```python
from build123d import *

# Parameters (mm, degrees)
SKETCH1_R           = 18
SKETCH1_R_2         = 2.1
SKETCH1_W           = 10.3
SKETCH1_H           = 10.3
BOSS_EXTRUDE1_DEPTH = 57
CUT_EXTRUDE4_DEPTH  = 40
SKETCH6_R           = 1.5
CUT_EXTRUDE5_DEPTH  = 36
SKETCH7_R           = 3
CUT_EXTRUDE6_DEPTH  = 3
CUT_EXTRUDE7_DEPTH  = 4
CHAMFER1_SIZE       = 1
CHAMFER1_SIZE2      = 2.747477419
CUT_EXTRUDE9_DEPTH  = 6
CHAMFER2_SIZE       = 0.5
CHAMFER2_SIZE2      = 1.37373871
CUT_EXTRUDE10_DEPTH = 35
CUT_EXTRUDE11_DEPTH = 58
CHAMFER3_SIZE       = 0.5
CHAMFER3_SIZE2      = 1.37373871
CUT_EXTRUDE13_DEPTH = 2


with BuildPart() as part:
    # Sketch1 → Boss-Extrude1 (new body)
    with BuildSketch(Plane(origin=(0, 0, 0), x_dir=(1, 0, 0), z_dir=(0, 1, 0))):
        Circle(SKETCH1_R)
        with Locations((13, 0)):
            Circle(SKETCH1_R_2, mode=Mode.SUBTRACT)
        with Locations((-13, 0)):
            Circle(SKETCH1_R_2, mode=Mode.SUBTRACT)
        Rectangle(SKETCH1_W, SKETCH1_H, mode=Mode.SUBTRACT)
    extrude(amount=BOSS_EXTRUDE1_DEPTH)

    # Sketch5 → Cut-Extrude4 (cut)
    with BuildSketch(Plane(origin=(0, 57, 0), x_dir=(1, 0, 0), z_dir=(0, 1, 0))):
        with BuildLine():
            Line((5.916079783, 17), (-5.916079783, 17))
            ThreePointArc((-5.916079783, 17), (0, 18), (5.916079783, 17))
        make_face()
        with BuildLine():
            Line((5.916079783, -17), (-5.916079783, -17))
            ThreePointArc((-5.916079783, -17), (0, -18), (5.916079783, -17))
        make_face()
    extrude(amount=-CUT_EXTRUDE4_DEPTH, mode=Mode.SUBTRACT)

    # Sketch6 → Cut-Extrude5 (cut, through all)
    with BuildSketch(Plane(origin=(0, 0, -17), x_dir=(-1, 0, 0), z_dir=(0, 0, -1))):
        with Locations((0, 47)):
            Circle(SKETCH6_R)
        with Locations((0, 22)):
            Circle(SKETCH6_R)
    extrude(amount=-CUT_EXTRUDE5_DEPTH, mode=Mode.SUBTRACT)

    # Sketch7 → Cut-Extrude6 (cut)
    with BuildSketch(Plane(origin=(0, 0, -17), x_dir=(-1, 0, 0), z_dir=(0, 0, -1))):
        with Locations((0, 47)):
            Circle(SKETCH7_R)
        with Locations((0, 22)):
            Circle(SKETCH7_R)
    extrude(amount=-CUT_EXTRUDE6_DEPTH, mode=Mode.SUBTRACT)

    # Sketch8 → Cut-Extrude7 (cut)
    with BuildSketch(Plane.XY.offset(17)):
        Polygon((0, 43.8), (2.771281292, 45.4), (2.771281292, 48.6), (0, 50.2), (-2.771281292, 48.6), (-2.771281292, 45.4), align=None)
        Polygon((0, 18.8), (2.771281292, 20.4), (2.771281292, 23.6), (0, 25.2), (-2.771281292, 23.6), (-2.771281292, 20.4), align=None)
    extrude(amount=-CUT_EXTRUDE7_DEPTH, mode=Mode.SUBTRACT)

    # Chamfer1
    chamfer1_edges = [part.edges().sort_by_distance(p)[0] for p in [
        (0, 57, -5.15),
        (-5.15, 57, 0),
        (0, 57, 5.15),
        (5.15, 57, 0),
    ]]
    chamfer1_side = [part.faces().sort_by_distance(p)[0] for p in [
        (14.267618119, 57, 10.141691708),
    ]]
    chamfer(chamfer1_edges, length=CHAMFER1_SIZE, length2=CHAMFER1_SIZE2, reference=chamfer1_side[0])

    # Sketch9 → Cut-Extrude9 (cut)
    with BuildSketch(Plane.XZ):
        with BuildLine():
            Line((15.438263477, -3.358179747), (9.406640719, -2.076118753))
            ThreePointArc((9.406640719, -2.076118753), (13.862833517, 4.059312543), (15.438263477, -3.358179747))
        make_face()
        with BuildLine():
            Line((-9.458796565, -2.163880365), (-15.354920877, -3.417140276))
            ThreePointArc((-15.354920877, -3.417140276), (-13.862833517, 4.059312543), (-9.458796565, -2.163880365))
        make_face()
    extrude(amount=-CUT_EXTRUDE9_DEPTH, mode=Mode.SUBTRACT)

    # Chamfer2
    chamfer2_edges = [part.edges().sort_by_distance(p)[0] for p in [
        (13.862833517, 0, 4.059312543),
        (12.422452098, 0, -2.71714925),
        (-13.862833517, 0, 4.059312543),
        (-12.406858721, 0, -2.79051032),
    ]]
    chamfer2_side = [part.faces().sort_by_distance(p)[0] for p in [
        (-17.490883118, 0, 0),
    ]]
    chamfer(chamfer2_edges, length=CHAMFER2_SIZE, length2=CHAMFER2_SIZE2, reference=chamfer2_side[0])

    # Sketch10 → Cut-Extrude10 (cut)
    with BuildSketch(Plane(origin=(0, 57, 0), x_dir=(1, 0, 0), z_dir=(0, 1, 0))):
        with BuildLine():
            Line((13, 4.2), (21, 4.2))
            Line((21, 4.2), (21, -4.2))
            Line((21, -4.2), (13, -4.2))
            ThreePointArc((13, -4.2), (8.8, 0), (13, 4.2))
        make_face()
        with BuildLine():
            Line((-13, 4.2), (-21, 4.2))
            Line((-21, 4.2), (-21, -4.2))
            Line((-21, -4.2), (-13, -4.2))
            ThreePointArc((-13, -4.2), (-8.8, 0), (-13, 4.2))
        make_face()
    extrude(amount=-CUT_EXTRUDE10_DEPTH, mode=Mode.SUBTRACT)

    # Sketch11 → Cut-Extrude11 (cut, through all)
    with BuildSketch(Plane.XZ):
        Polygon((-14.185073919, 7.986468426), (-10.328348261, 12.582735084), (-8.796259375, 11.297159865), (-12.652985033, 6.700893206), align=None)
    extrude(amount=-CUT_EXTRUDE11_DEPTH, mode=Mode.SUBTRACT)

    # Chamfer3
    chamfer3_edges = [part.edges().sort_by_distance(p)[0] for p in [
        (-13.419029476, 0, 7.343680816),
        (-10.724622204, 0, 8.999026536),
        (-9.562303818, 0, 11.939947475),
        (-12.25671109, 0, 10.284601755),
    ]]
    chamfer3_side = [part.faces().sort_by_distance(p)[0] for p in [
        (-17.949088312, 0, 0),
    ]]
    chamfer(chamfer3_edges, length=CHAMFER3_SIZE, length2=CHAMFER3_SIZE2, reference=chamfer3_side[0])

    # Sketch13 → Cut-Extrude13 (cut)
    with BuildSketch(Plane(origin=(0, 57, 0), x_dir=(1, 0, 0), z_dir=(0, 1, 0))):
        with BuildLine():
            Line((-8.796259375, -11.297159865), (-8.796259375, 15.704324914))
            ThreePointArc((-8.796259375, 15.704324914), (-11.720909208, 13.660903606), (-14.185073919, 11.080779662))
            Line((-14.185073919, 11.080779662), (-14.185073919, -7.986468426))
            Line((-14.185073919, -7.986468426), (-8.796259375, -11.297159865))
        make_face()
    extrude(amount=-CUT_EXTRUDE13_DEPTH, mode=Mode.SUBTRACT)


solid = part.part
```
Part model, mm, in its own coordinate system. A direction names the side the tool comes from. Round coordinates to 2 decimals unless told otherwise and drop trailing zeros. Order: outer loops, then holes, each group sorted by start corner. A loop starts at its lowest first (then second) coordinate and runs counter-clockwise, first axis right, second up. Notation, with made-up numbers: M -15,22.25 L -1,22.25 A15 cw -1,38.25 Z; hole C 9.5,25 d11. An arc over 180 degrees is marked long. Answer in a Markdown table with one row per item. Add a question column.
Q1. Cut at C-C on y = 47. Give the number of separate pieces and of enclosed holes in the cut face, and give its area (3 significant figures).
Q2. Pin check, flat tips, straight feed: pin 1 (1 mm diameter, centred on y = 47, z = 15, fed in from -X); pin 2 (6.5 mm diameter, centred on x = -13, z = 0, fed in from +Y); pin 3 (6 mm diameter, centred on x = 1, y = 47, fed in from +Z). Stop position of each tip, or through.
Q3. Cut at A-A on z = 14. Give the cut face in (x, y).
Q4. Wall check: L1, parallel to Y at x = 0, z = -11; L2, parallel to Z at x = 2.5, y = 38.5; L3, parallel to Z at x = -12, y = 38.5. Give the ranges that are in metal, low to high. Write a range as from..to.
Q5. 3-axis set-ups, long thin cutter, end or side, ignore diameter. For faces 4 (the face through (0, 37, -17)), 5 (the face through (1.37, 44.59, 15.03)), 6 (the face through (12.416, 0.696, -2.968)), 7 (the face through (8.8, 39.7, 0.1)): which of +Z, -Z, +X, -X, +Y, -Y reach the whole face in a straight line?
Q6. Cut at B-B on y = 33.5. Give the cut face in (x, z).
Q7. Mould opens along Z. For faces 1 (the face through (8, 0, 0)), 2 (the face through (-1.3, 45.6, 13)), 3 (the face through (-15.1, 13.89, -0.09)) say: +Z half, -Z half, draft (parallel to the pull), parting line (faces both ways), or undercut.
Q8. Cut at D-D on z = -13. Give the cut face in (x, y).
Established:
| question | item | result |
|---|---|---|
| 1 | separate pieces | 2 |
| 1 | enclosed holes | 1 |
| 1 | area | 657 mm2 |
| 2 | pin 1 | stops at x = -10.67 |
| 2 | pin 2 | stops at y = 22 |
| 2 | pin 3 | stops at z = 17 |
| 3 | outline | M -11.31,0 L 11.31,0 L 11.31,57 L -11.31,57 Z; hole M -2.77,20.4 L 0,18.8 L 2.77,20.4 L 2.77,23.6 L 0,25.2 L -2.77,23.6 Z; hole M -2.77,45.4 L 0,43.8 L 2.77,45.4 L 2.77,48.6 L 0,50.2 L -2.77,48.6 Z |
| 4 | L1 | y = 0..20.5, 23.5..45.5, 48.5..57 |
| 4 | L2 | z = -17..-5.15, 5.15..17 |
| 4 | L3 | z = -13.42..-4.08, 4.08..7.48, 10.59..13.42 |
| 5 | face 4 | -Z, +X, -X, +Y |
| 5 | face 5 | +Z |
| 5 | face 6 | -Y |
| 5 | face 7 | +X, +Y |
| 6 | outline | M -17.5,-4.2 A18 ccw -5.92,-17 L 5.92,-17 A18 ccw 17.5,-4.2 L 13,-4.2 A4.2 cw 13,4.2 L 17.5,4.2 A18 ccw 5.92,17 L -5.92,17 A18 ccw -17.5,4.2 L -13,4.2 A4.2 cw -13,-4.2 Z; hole M -14.19,7.99 L -12.65,6.7 L -8.8,11.3 L -10.33,12.58 Z; hole M -5.15,-5.15 L 5.15,-5.15 L 5.15,5.15 L -5.15,5.15 Z |
| 7 | face 1 | draft |
| 7 | face 2 | +Z half |
| 7 | face 3 | undercut |
| 8 | outline | M -12.45,0 L 12.45,0 L 12.45,57 L -8.8,57 L -8.8,55 L -12.45,55 Z; hole C 0,22 d3; hole C 0,47 d3 |
